```python
from build123d import *

# Parameters (mm, degrees)
F0_R     = 13
F0_R_2   = 13.1
F1_DEPTH = 8


with BuildPart() as f1:
    # F0 (on Top) → F1 (new body)
    with BuildSketch(Plane.XY):
        Polygon((-46.768434, 13.382968), (-51, 0), (-46.768434, -13.382968), (0, -23.456169), (46.768434, -13.382968), (51, 0), (46.768434, 13.382968), (0, 23.456169), align=None)
        with Locations((-31.9, 0)):
            Circle(F0_R, mode=Mode.SUBTRACT)
        Circle(F0_R_2, mode=Mode.SUBTRACT)
        with Locations((31.9, 0)):
            Circle(F0_R, mode=Mode.SUBTRACT)
    extrude(amount=F1_DEPTH)


solid = f1.part
```
Read the model definition and answer for the solid it produces. Units are mm, in the model's axes. Give positions to 0.01 mm unless a question says otherwise; leave off trailing zeros. Write each loop counter-clockwise with the first axis right and the second up, starting at its lowest first coordinate (ties: lowest second). Pieces come first, ordered by that corner, then holes. Notation, with made-up numbers: M 31.25,72 L 78.25,72 A7 cw 78.25,82 Z; hole C 51,86 d2. An arc over 180 degrees is marked long. Put each result on its own line as item: value. Start each with the question number.
1. Consider line 1 along Y through (x, z) = (0, 3.5); line 2 along X through (y, z) = (-11, 3); line 3 along X through (y, z) = (-7, 2). Determine where each line is inside the solid, lowest interval first.
2. The part is cut by section D-D, the plane y = -19. Give the vertices of the cut face in (x, z).
3. The part is cut by section A-A, the plane z = 5.75. Give the vertices of the cut face in (x, y), and give its area (3 significant figures).
4. The part is cut by section C-C, the plane x = -31.9. Give the vertices of the cut face in (y, z).
5. The part is cut by section B-B, the plane x = -1. Give the vertices of the cut face in (y, z).
6. For a pull along X with two mould halves and no side action, classify faces 1 (the flat face through (-23.06, 18.49, 3.94)), 2 (the flat face through (48.855, -6.785, 3.944)), 3 (the cylindrical face through (-19.5, 3.9, 3.9)) as released by +X, released by -X, zero draft, split by the parting line, or undercut.
7. Each of these flat-tipped pins is pushed along its axis until it touches: pin 1 Ø2 at (y, z) = (-11, 6.5) entering from -X; pin 2 Ø21 at (x, y) = (31.9, 0) entering from -Z; pin 3 Ø3 at (x, z) = (-27.5, 2.5) entering from +Y. Where does it stop, or does it pass through?
Final values:
1. line 1: y = -23.46 to -13.1, 13.1 to 23.46
1. line 2: x = -47.52 to -38.83, -24.97 to -7.11, 7.11 to 24.97, 38.83 to 47.52
1. line 3: x = -48.79 to -42.85, -20.95 to -11.07, 11.07 to 20.95, 42.85 to 48.79
2. outline: M -20.69,0 L 20.69,0 L 20.69,8 L -20.69,8 Z
3. outline: M -51,0 L -46.77,-13.38 L 0,-23.46 L 46.77,-13.38 L 51,0 L 46.77,13.38 L 0,23.46 L -46.77,13.38 Z; hole C -31.9,0 d26; hole C 0,0 d26.2; hole C 31.9,0 d26
3. area: 1,960 mm²
4. outline: M -16.59,0 L -13,0 L -13,8 L -16.59,8 Z; M 13,0 L 16.59,0 L 16.59,8 L 13,8 Z
5. outline: M -23.24,0 L -13.06,0 L -13.06,8 L -23.24,8 Z; M 13.06,0 L 23.24,0 L 23.24,8 L 13.06,8 Z
6. face 1: released by -X
6. face 2: released by +X
6. face 3: undercut
7. pin 1: stops at x = -47.84
7. pin 2: passes through
7. pin 3: stops at y = 17.86
